Verification items for the finished model (mm, model axes). Give positions to 0.01 mm unless a question says otherwise; leave off trailing zeros. Loops run counter-clockwise (first coordinate to the right, second up) from the corner with the lowest first, then second, coordinate; pieces in that order, holes last. Notation, with made-up numbers: M -2.5,55 L 13.5,55 A22 ccw 13.5,67 Z; hole C 46,18.25 d8. An arc over 180 degrees is marked long. Put each result on its own line as item: value. Start each with the question number.
from build123d import *

# Parameters (mm, degrees)
F1_DEPTH = 17.9832
F2_R     = 152.4
F3_R     = 3.302
F4_R     = 5.08


with BuildPart() as f1:
    # F0 (on Top) → F1 (new body)
    with BuildSketch(Plane.XY):
        Polygon((-123.825, -698.5), (-123.825, -717.55), (0, -717.55), (0, 0), (-850.9, 0), (-850.9, -304.8), (-171.45, -304.8), (-171.45, -698.5), align=None)
    extrude(amount=F1_DEPTH)

    # F2
    f2_edges = [f1.edges().sort_by_distance(p)[0] for p in [
        (-171.45, -304.8, 8.9916),
    ]]
    fillet(f2_edges, radius=F2_R)

    # F3
    f3_edges = [f1.edges().sort_by_distance(p)[0] for p in [
        (-123.825, -698.5, 8.9916),
    ]]
    fillet(f3_edges, radius=F3_R)

    # F4
    f4_edges = [f1.edges().sort_by_distance(p)[0] for p in [
        (-171.45, -577.85, 17.9832),
    ]]
    fillet(f4_edges, radius=F4_R)


solid = f1.part
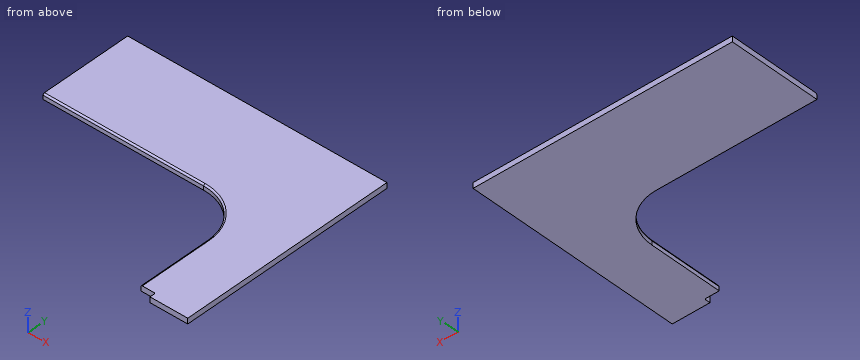
Q1. Scan lines: L1, parallel to Y at x = -786, z = 8.5; L2, parallel to X at y = -549.5, z = 13.25; L3, parallel to Y at x = -574.5, z = 15.75. Record each from-to range of solid material in increasing order.
Q2. Cross-section at A-A, the plane z = 2.75. Record the boundary of the cut face in (x, y) (3 decimals).
Q3. Go/stop test with flat-tipped pins: pin 1 (8 mm diameter, centred on y = -712.5, z = 13.5, fed in from -X) (3 decimals); pin 2 (2 mm diameter, centred on x = -495, z = 3, fed in from -Y); pin 3 (10.5 mm diameter, centred on y = -547.5, z = 5.5, fed in from -X). Record where each tip stops, or that it passes through.
Q4. Cross-section at B-B, the plane y = -600. Record the boundary of the cut face in (x, z), then the cut area to 3 significant figures.
Ans:
1. L1: y = -304.8 to 0
1. L2: x = -171.44 to 0
1. L3: y = -303.93 to 0
2. outline: M -850.9,-304.8 L -323.85,-304.8 A152.4 cw -171.45,-457.2 L -171.45,-698.5 L -127.127,-698.5 A3.302 cw -123.825,-701.802 L -123.825,-717.55 L 0,-717.55 L 0,0 L -850.9,0 Z
3. pin 1: stops at x = -123.825
3. pin 2: stops at y = -304.8
3. pin 3: stops at x = -171.45
4. outline: M -171.45,0 L 0,0 L 0,17.98 L -166.37,17.98 A5.08 ccw -171.45,12.9 Z
4. area: 3,080 mm^2
